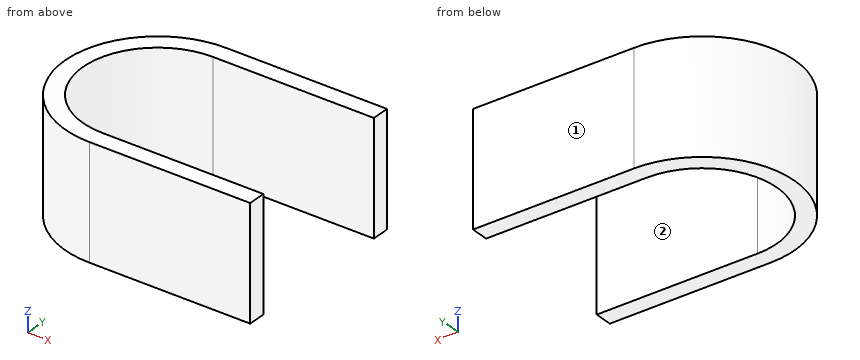
from build123d import *

# Parameters (mm, degrees)
BOSS_EXTRUDE1_DEPTH = 28


with BuildPart() as part:
    # Sketch1 → Boss-Extrude1 (new body)
    with BuildSketch(Plane.XY):
        with BuildLine():
            ThreePointArc((0, 22.9), (7.09788701, 21.772230019), (13.496666255, 18.5))
            Line((13.496666255, 18.5), (40, 18.5))
            Line((40, 18.5), (40, 22.9))
            Line((40, 22.9), (0, 22.9))
        make_face()
        with BuildLine():
            ThreePointArc((0, -18.5), (-18.5, 0), (0, 18.5))
            Line((0, 18.5), (13.496666255, 18.5))
            ThreePointArc((13.496666255, 18.5), (7.09788701, 21.772230019), (0, 22.9))
            ThreePointArc((0, 22.9), (-22.9, 0), (0, -22.9))
            ThreePointArc((0, -22.9), (7.09788701, -21.772230019), (13.496666255, -18.5))
            Line((13.496666255, -18.5), (0, -18.5))
        make_face()
        with BuildLine():
            Line((40, -18.5), (13.496666255, -18.5))
            ThreePointArc((13.496666255, -18.5), (7.09788701, -21.772230019), (0, -22.9))
            Line((0, -22.9), (40, -22.9))
            Line((40, -22.9), (40, -18.5))
        make_face()
    extrude(amount=BOSS_EXTRUDE1_DEPTH)


solid = part.part
Can you work these out from the model? Positions are in its coordinate system, mm. Face numbers are marked on the shaded views. A direction names the side the tool comes from. Round coordinates to 2 decimals unless told otherwise and drop trailing zeros. Loops run counter-clockwise (first coordinate to the right, second up) from the corner with the lowest first, then second, coordinate; pieces in that order, holes last. Notation, with made-up numbers: (62.5, 54) - (80.5, 54) arc R8 cw to (80.5, 69) - close; hole circle Ø6 at (-4, 26.5). An arc over 180 degrees is marked (long way). Write item = value, one per line. Start each with the question number.
(1) If we section it at D-D (y = 6): Please give me the cut outline in (x, z).
(2) If we section it at B-B (x = -10.5): Please give me the cut outline in (y, z), and give its area (3 significant figures).
(3) If I drill on probe 1 along Y at (x, z) = (5, 1.5); probe 2 along X at (y, z) = (0, 12.75); probe 3 along Y at (x, z) = (-9, 4.75), over which ranges is the centre line in solid material (lowest first)? Write a range as [from, to].
(4) For the marked faces 1 and 2, which set-ups out of +Z, -Z, +X, -X, +Y, -Y let a thin tool reach every point of the face, with its end or its side?
(5) For P1, Ø1.5, axis at x = -8.5, z = 22.5, coming from the -Y side; P2, Ø12, axis at x = -16, y = 11, coming from the -Z side; P3, Ø6, axis at y = 13, z = 11.5, coming from the +X side; P4, Ø12, axis at y = 3.5, z = 21, coming from the -X side, each with a flat end and sliding along its axis, tell me the tip position at first contact or that it passes through.
(6) If we section it at A-A (z = 14.5): Please give me the cut outline in (x, y).
(7) If we section it at C-C (y = 0): Please give me the cut outline in (x, z), and give its area (3 significant figures).
Ans:
q1.outline = (-22.1, 0) - (-17.5, 0) - (-17.5, 28) - (-22.1, 28) - close
q2.outline = (-20.35, 0) - (-15.23, 0) - (-15.23, 28) - (-20.35, 28) - close; (15.23, 0) - (20.35, 0) - (20.35, 28) - (15.23, 28) - close
q2.area = 287 mm²
q3.probe_1 = [-22.9, -18.5], [18.5, 22.9]
q3.probe_2 = [-22.9, -18.5]
q3.probe_3 = [-21.06, -16.16], [16.16, 21.06]
q4.face_1 = +Z, -Z, +X, -X, +Y
q4.face_2 = +Z, -Z, +X
q5.P1 = -21.55
q5.P2 = 0
q5.P3 = -9.29
q5.P4 = -22.9
q6.outline = (0, -22.9) - (40, -22.9) - (40, -18.5) - (0, -18.5) arc R18.5 cw to (0, 18.5) - (40, 18.5) - (40, 22.9) - (0, 22.9) arc R22.9 ccw to start
q7.outline = (-22.9, 0) - (-18.5, 0) - (-18.5, 28) - (-22.9, 28) - close
q7.area = 123 mm²
